Could you check a few things on this drawing? It's one solid part, dimensions in mm from its lowest x, y, z. Give positions to 0.01 mm unless a question says otherwise; leave off trailing zeros. Loops run counter-clockwise (first coordinate to the right, second up) from the corner with the lowest first, then second, coordinate; pieces in that order, holes last. Notation, with made-up numbers: (75.25, 57) - (123.25, 57) arc R31 cw to (123.25, 93) - close; hole circle Ø8 at (-8.75, -13). An arc over 180 degrees is marked (long way). Answer as a JSON object with one key per item and string values.
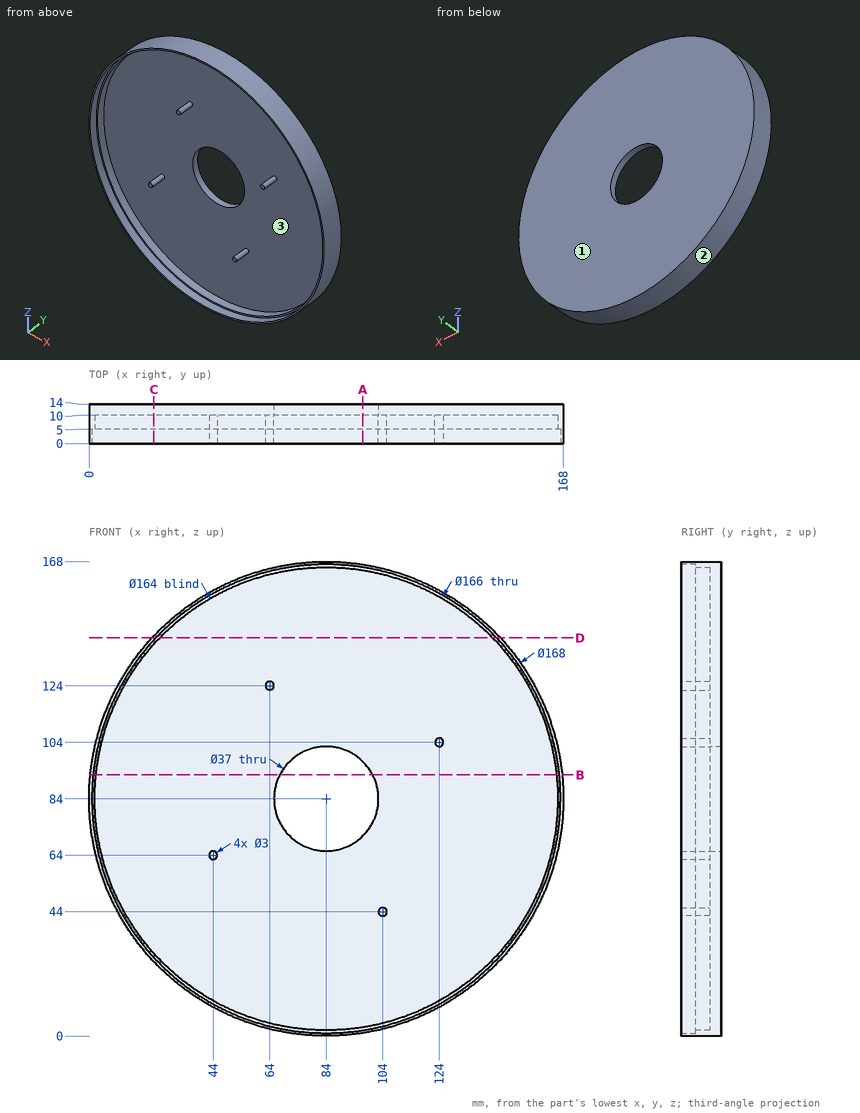
1) Imagine slicing it at C-C on x = 23. Write out the boundary of the cut face in (y, z).
Check sheet entries:
{"outline": "(0, 26.25) - (14, 26.25) - (14, 141.75) - (0, 141.75) - (0, 140.28) - (5, 140.28) - (5, 138.8) - (10, 138.8) - (10, 29.2) - (5, 29.2) - (5, 27.72) - (0, 27.72) - close"}
2) If we mould it in two halves opening along Z, with no side actions, what happens to the marked faces 1, 2 and 3? For each: released by +Z, released by -Z, zero draft, split by the parting line, or undercut.
Check sheet entries:
{"face 1": "zero draft", "face 2": "split by the parting line", "face 3": "undercut"}
3) Imagine slicing it at A-A on x = 97. Write out the boundary of the cut face in (y, z), and give its area (3 significant figures).
Check sheet entries:
{"outline": "(0, 1.01) - (14, 1.01) - (14, 70.84) - (10, 70.84) - (10, 3.04) - (5, 3.04) - (5, 2.02) - (0, 2.02) - close; (0, 165.98) - (5, 165.98) - (5, 164.96) - (10, 164.96) - (10, 97.16) - (14, 97.16) - (14, 166.99) - (0, 166.99) - close", "area": "589 mm2"}
4) I need wall thicknesses on L1, parallel to X at y = 11.45, z = 84; L2, parallel to X at y = 6.5, z = 84; L3, parallel to Y at x = 110.5, z = 32. Which ranges of each line are inside material? Lowest first, please.
Check sheet entries:
{"L1": "0 to 65.5, 102.5 to 168", "L2": "0 to 2, 166 to 168", "L3": "10 to 14"}
5) Imagine slicing it at D-D on z = 141. Write out the boundary of the cut face in (x, y).
Check sheet entries:
{"outline": "(22.3, 0) - (23.67, 0) - (23.67, 5) - (25.05, 5) - (25.05, 10) - (142.95, 10) - (142.95, 5) - (144.33, 5) - (144.33, 0) - (145.7, 0) - (145.7, 14) - (22.3, 14) - close"}
6) I'm going to push flat-ended pins straight in: P1, Ø6, axis at y = 6.5, z = 139, coming from the -X side; P2, Ø8, axis at y = 7.5, z = 77.5, coming from the +X side; P3, Ø8, axis at y = 2, z = 120, coming from the -X side. Where does each tip first touch, or does it pass through?
Check sheet entries:
{"P1": "x = 18.03", "P2": "x = 167.96", "P3": "x = 6.33"}
7) Imagine slicing it at B-B on z = 92.5. Write out the boundary of the cut face in (x, y), and give its area (3 significant figures).
Check sheet entries:
{"outline": "(0.43, 0) - (1.44, 0) - (1.44, 5) - (2.44, 5) - (2.44, 10) - (67.57, 10) - (67.57, 14) - (0.43, 14) - close; (100.43, 10) - (165.56, 10) - (165.56, 5) - (166.56, 5) - (166.56, 0) - (167.57, 0) - (167.57, 14) - (100.43, 14) - close", "area": "567 mm2"}
